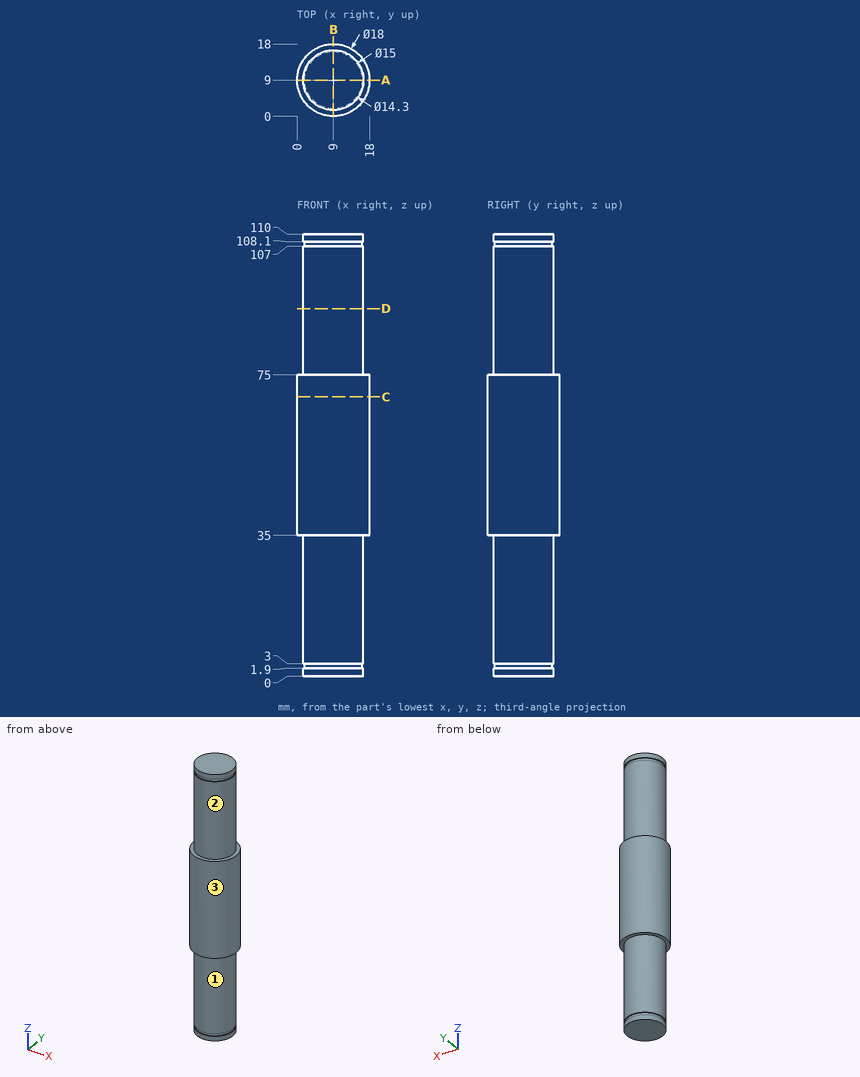
Can you work these out from the drawing? Everything is in mm from the part's minimum corner. A direction names the side the tool comes from. Give positions to 0.01 mm unless a question says otherwise; leave off trailing zeros. Loops run counter-clockwise (first coordinate to the right, second up) from the corner with the lowest first, then second, coordinate; pieces in that order, holes last. Notation, with made-up numbers: (29.25, 53) -> (87.25, 53) arc R16 cw to (87.25, 71) -> close; hole circle Ø5 at (-16.5, 87). An arc over 180 degrees is marked (long way). Return JSON: item names as keys, results as strings.
Item 1: I need wall thicknesses on L1, parallel to Z at x = 1.25, y = 7.5; L2, parallel to Y at x = 8.5, z = 28; L3, parallel to X at y = 8.5, z = 71. Which ranges of each line are inside material? Lowest first, please. Write a range as from..to.
Geometry results:
{"L1": "z = 35..75", "L2": "y = 1.52..16.48", "L3": "x = 0.01..17.99"}
Item 2: If we section it at C-C on z = 69.5: List the corners of the cut face in (x, y) for me, plus the area to 3 significant figures.
Geometry results:
{"outline": "circle Ø18 at (9, 9)", "area": "254 mm²"}
Item 3: I'm going to push flat-ended pins straight in: pin 1 (3 mm diameter, centred on y = 5.5, z = 48.5, fed in from +X); pin 2 (9 mm diameter, centred on x = 9.5, y = 13, fed in from -Z); pin 3 (3 mm diameter, centred on y = 13, z = 63.5, fed in from +X); pin 4 (3 mm diameter, centred on y = 15, z = 33, fed in from -X). Where does each tip first touch, or does it pass through?
Geometry results:
{"pin 1": "stops at x = 17.77", "pin 2": "stops at z = 0", "pin 3": "stops at x = 17.65", "pin 4": "stops at x = 3"}
Item 4: If we section it at A-A on y = 9: List the corners of the cut face in (x, z) for me, plus the area to 3 significant figures.
Geometry results:
{"outline": "(0, 35) -> (1.5, 35) -> (1.5, 3) -> (1.85, 3) -> (1.85, 1.9) -> (1.5, 1.9) -> (1.5, 0) -> (16.5, 0) -> (16.5, 1.9) -> (16.15, 1.9) -> (16.15, 3) -> (16.5, 3) -> (16.5, 35) -> (18, 35) -> (18, 75) -> (16.5, 75) -> (16.5, 107) -> (16.15, 107) -> (16.15, 108.1) -> (16.5, 108.1) -> (16.5, 110) -> (1.5, 110) -> (1.5, 108.1) -> (1.85, 108.1) -> (1.85, 107) -> (1.5, 107) -> (1.5, 75) -> (0, 75) -> close", "area": "1,770 mm²"}
Item 5: Which directions (+Z, -Z, +X, -X, +Y, -Y) give clear straight access to the entire face, cutting with the end or side of a thin tool? Please do the marked faces 1, 2 and 3.
Geometry results:
{"face 1": "-Z", "face 2": "+Z", "face 3": "+Z, -Z"}
Item 6: If we section it at D-D on z = 91.5: List the corners of the cut face in (x, y) for me, plus the area to 3 significant figures.
Geometry results:
{"outline": "circle Ø15 at (9, 9)", "area": "177 mm²"}
